Could you check a few things on this model? Use its own coordinates, in mm. A direction names the side the tool comes from. Coordinates: 2 decimals unless noted, no trailing zeros. Loops run counter-clockwise (first coordinate to the right, second up) from the corner with the lowest first, then second, coordinate; pieces in that order, holes last. Notation, with made-up numbers: M 38,87.25 L 86,87.25 A27 ccw 86,121.25 Z; hole C -22,69.5 d7. An arc over 180 degrees is marked long. Return JSON: item names as keys, results as strings. Group by question number.
from build123d import *

# Parameters (mm, degrees)
SKETCH1_W               = 2.032
SKETCH1_H               = 25.146
CUT_EXTRUDE1_REACH      = 26.41
CUT_EXTRUDE1_END_RADIUS = 1.524
SKETCH2_W               = 0.508
SKETCH2_H               = 0.889
CIRPATTERN1_COUNT       = 16
SKETCH3_R               = 3.556
SKETCH3_R_2             = 1.524
BOSS_EXTRUDE1_DEPTH     = 6.35
BOSS_EXTRUDE2_START     = 6.35
SKETCH4_R               = 17.78
SKETCH4_R_2             = 1.524
BOSS_EXTRUDE2_DEPTH     = 6.35
CUT_EXTRUDE2_REACH      = 47.438
SKETCH11_R              = 1.63195
CIRPATTERN2_COUNT       = 6
CHAMFER1_SIZE           = 3.048
CHAMFER1_SIZE2          = 5.279290861
SKETCH13_R              = 11.43
SKETCH13_R_2            = 6.54812
BOSS_EXTRUDE4_DEPTH     = 12.7
FILLET4_R               = 0.254
CHAMFER2_SIZE           = 0.851662
CHAMFER2_SIZE2          = 0.83947
BOSS_EXTRUDE5_START     = -6.35
SKETCH15_R              = 4.699
SKETCH15_R_2            = 3.556
BOSS_EXTRUDE5_DEPTH     = 6.35


with BuildPart() as part:
    # Sketch1 → Revolve2 (revolve)
    with BuildSketch(Plane.XY, mode=Mode.PRIVATE) as revolve2_sk:
        with Locations((-2.54, 10.505774136)):
            Rectangle(SKETCH1_W, SKETCH1_H)
    revolve(revolve2_sk.sketch.rotate(Axis((0, 8.215698649, 0), (0, -1, 0)), 270), axis=Axis((0, 8.215698649, 0), (0, -1, 0)))

    # Cut-Extrude1: up to this cylinder (the profile starts outside it)
    cut_extrude1_end = Plane(origin=(0, -0.733726, 0), z_dir=(0, 1, 0)) * Cylinder(CUT_EXTRUDE1_END_RADIUS, 56.868, mode=Mode.PRIVATE)
    # Sketch2 → Cut-Extrude1 (cut, up to the surface)
    with BuildSketch(Plane.ZY.offset(3.556), mode=Mode.PRIVATE) as cut_extrude1_sk1:
        with Locations((0.000240101, -0.733725864)):
            Rectangle(SKETCH2_W, SKETCH2_H)
    cut_extrude1_tool1 = extrude(cut_extrude1_sk1.sketch, amount=-CUT_EXTRUDE1_REACH, mode=Mode.PRIVATE) - cut_extrude1_end
    cut_extrude1 = cut_extrude1_tool1.solids().sort_by_distance((-3.556, -0.733726, 0.00024))[0]
    add(cut_extrude1, mode=Mode.SUBTRACT)

    # CirPattern1: Cut-Extrude1 ×16 about axis
    cirpattern1_axis = Axis((0, 0, 0), (0, 1, 0))
    for i in range(1, CIRPATTERN1_COUNT):
        add(cut_extrude1.rotate(cirpattern1_axis, i * 360 / CIRPATTERN1_COUNT), mode=Mode.SUBTRACT)

    # Sketch3 → Boss-Extrude1 (add)
    with BuildSketch(Plane(origin=(0, 23.078774136, 0), x_dir=(-1, 0, 0), z_dir=(0, -1, 0))):
        with Locations(Location((0, 0, 0), (0, 0, 270))):
            Circle(SKETCH3_R)
        with Locations(Location((0, 0, 0), (0, 0, 270))):
            Circle(SKETCH3_R_2, mode=Mode.SUBTRACT)
    extrude(amount=-BOSS_EXTRUDE1_DEPTH)

    # Sketch4 → Boss-Extrude2 (add)
    with BuildSketch(Plane(origin=(0, 29.428774136, 0), x_dir=(1, 0, 0), z_dir=(0, 1, 0)).offset(BOSS_EXTRUDE2_START)):
        with Locations(Location((0, 0, 0), (0, 0, 270))):
            Circle(SKETCH4_R)
        with Locations(Location((0, 0, 0), (0, 0, 270))):
            Circle(SKETCH4_R_2, mode=Mode.SUBTRACT)
    extrude(amount=-BOSS_EXTRUDE2_DEPTH)

    # Sketch11 → Cut-Extrude2 (cut, up to next)
    with BuildSketch(Plane(origin=(0, 35.778774136, 0), x_dir=(1, 0, 0), z_dir=(0, 1, 0)), mode=Mode.PRIVATE) as cut_extrude2_sk1:
        with Locations(Location((0, -15.24, 0), (0, 0, 270))):
            Circle(SKETCH11_R)
    cut_extrude2_tool1 = extrude(cut_extrude2_sk1.sketch, amount=-CUT_EXTRUDE2_REACH, mode=Mode.PRIVATE) & part.part
    cut_extrude2 = cut_extrude2_tool1.solids().sort_by_distance((0, 35.778774, 15.24))[0]
    add(cut_extrude2, mode=Mode.SUBTRACT)

    # CirPattern2: Cut-Extrude2 ×6 about axis
    cirpattern2_axis = Axis((0, 0, 0), (0, 1, 0))
    for i in range(1, CIRPATTERN2_COUNT):
        add(cut_extrude2.rotate(cirpattern2_axis, i * 360 / CIRPATTERN2_COUNT), mode=Mode.SUBTRACT)

    # Chamfer1
    chamfer1_edges = [part.edges().sort_by_distance(p)[0] for p in [
        (0, 35.778774136, -1.524),
    ]]
    chamfer1_side = [part.faces().sort_by_distance(p)[0] for p in [
        (0, 35.778774136, -17.277105657),
    ]]
    chamfer(chamfer1_edges, length=CHAMFER1_SIZE, length2=CHAMFER1_SIZE2, reference=chamfer1_side[0])

    # Sketch13 → Boss-Extrude4 (add)
    with BuildSketch(Plane(origin=(0, 35.778774136, 0), x_dir=(1, 0, 0), z_dir=(0, 1, 0))):
        with Locations(Location((0, 0, 0), (0, 0, 270))):
            Circle(SKETCH13_R)
        with Locations(Location((0, 0, 0), (0, 0, 270))):
            Circle(SKETCH13_R_2, mode=Mode.SUBTRACT)
    extrude(amount=BOSS_EXTRUDE4_DEPTH)

    # Fillet4
    fillet4_edges = [part.edges().sort_by_distance(p)[0] for p in [
        (0, 35.778774136, -11.43),
    ]]
    fillet(fillet4_edges, radius=FILLET4_R)

    # Chamfer2
    chamfer2_edges = [part.edges().sort_by_distance(p)[0] for p in [
        (0, 48.478774136, -6.54812),
    ]]
    chamfer2_side = [part.faces().sort_by_distance(p)[0] for p in [
        (0, 48.478774136, -11.10671078),
    ]]
    chamfer(chamfer2_edges, length=CHAMFER2_SIZE, length2=CHAMFER2_SIZE2, reference=chamfer2_side[0])

    # Sketch15 → Boss-Extrude5 (add)
    with BuildSketch(Plane(origin=(0, 29.428774136, 0), x_dir=(1, 0, 0), z_dir=(0, 1, 0)).offset(BOSS_EXTRUDE5_START)):
        with Locations(Location((0, 0, 0), (0, 0, 270))):
            Circle(SKETCH15_R)
        with Locations(Location((0, 0, 0), (0, 0, 270))):
            Circle(SKETCH15_R_2, mode=Mode.SUBTRACT)
    extrude(amount=BOSS_EXTRUDE5_DEPTH)


solid = part.part
(1) Imagine slicing it at D-D, the plane z = 12.5. Write out the boundary of the cut face in (x, y).
(2) Imagine slicing it at C-C, the plane y = 11.5. Write out the boundary of the cut face in (x, z), then the cut area to 3 significant figures.
(3) We'd pull the mould along X, two halves only. Please class faces 3 (the face through (-17.36, 32.65, -3.85)), 4 (the face through (4, 23.079, -1)), 5 (the face through (1, -0.289, -2.3)), 6 (the face through (2.4, -1.178, -1)): +X half, -X half, draft (parallel to the pull), parting line (faces both ways), or undercut.
(4) Imagine slicing it at A-A, the plane y = 32.5. Write out the boundary of the cut face in (x, z).
(5) Imagine slicing it at B-B, the plane z = -15.24. Write out the boundary of the cut face in (x, y), then the cut area to 3 significant figures.
(6) If I drill on L1, parallel to X at y = 33.5, z = -7.62; L2, parallel to Z at x = -13.5, y = 32.5; L3, parallel to X at y = 30.25, z = 0, over which ranges is the centre line in solid material (lowest first)? Write a range as [from, to].
(7) Will these pins go through, and if not, where does the flat tip stop? P1, Ø6, axis at y = 41, z = -11.5, coming from the -X side; P2, Ø1, axis at y = -1, z = 2.5, coming from the -X side; P3, Ø2, axis at x = -1.5, z = 2, coming from the +Y side.
(8) For faces 1 (the face through (-14.816, 32.648, 7.832)), 2 (the face through (1.62, -0.74, -1.98)), which set-ups out of +Z, -Z, +X, -X, +Y, -Y let a thin tool reach every point of the face, with its end or its side?
Checks:
{
 "1": {"outline": "M -12.64,29.43 L 12.64,29.43 L 12.64,35.78 L -12.64,35.78 Z"},
 "2": {"outline": "C 0,0 d7.11; hole C 0,0 d3.05", "area": "32.4 mm²"},
 "3": {"face 3": "parting line", "face 4": "draft", "face 5": "undercut", "face 6": "undercut"},
 "4": {"outline": "C 0,0 d35.56; hole C -13.2,-7.62 d3.26; hole C -13.2,7.62 d3.26; hole C 0,0 d5.36; hole C 0,-15.24 d3.26; hole C 0,15.24 d3.26; hole C 13.2,-7.62 d3.26; hole C 13.2,7.62 d3.26"},
 "5": {"outline": "M -9.16,29.43 L -1.63,29.43 L -1.63,35.78 L -9.16,35.78 Z; M 1.63,29.43 L 9.16,29.43 L 9.16,35.78 L 1.63,35.78 Z", "area": "95.6 mm²"},
 "6": {"L1": "[-16.06, -14.83], [-11.57, 11.57], [14.83, 16.06]", "L2": "[-11.57, -9.22], [-6.02, 6.02], [9.22, 11.57]", "L3": "[-17.78, -1.52], [1.52, 17.78]"},
 "7": {"P1": "x = -7.64", "P2": "x = -2.94", "P3": "y = 33.92"},
 "8": {"face 1": "+Y, -Y", "face 2": "none"}
}
